```python
from build123d import *

# Parameters (mm, degrees)
SKETCH1_W           = 127.75
SKETCH1_H           = 298.45
SKETCH1_R           = 4.95
BOSS_EXTRUDE1_DEPTH = 10
SKETCH4_R           = 2.5
CUT_EXTRUDE2_DEPTH  = 11


with BuildPart() as part:
    # Sketch1 → Boss-Extrude1 (new body)
    with BuildSketch(Plane(origin=(0, 0, 0), x_dir=(1, 0, 0), z_dir=(0, 1, 0))):
        with Locations((63.875, 149.225)):
            Rectangle(SKETCH1_W, SKETCH1_H)
        with Locations((19, 277)):
            Circle(SKETCH1_R, mode=Mode.SUBTRACT)
        with Locations((108.75, 277)):
            Circle(SKETCH1_R, mode=Mode.SUBTRACT)
        with Locations((108.75, 19)):
            Circle(SKETCH1_R, mode=Mode.SUBTRACT)
        with Locations((19, 19)):
            Circle(SKETCH1_R, mode=Mode.SUBTRACT)
        with Locations((19, 108)):
            Circle(SKETCH1_R, mode=Mode.SUBTRACT)
        with Locations((108.75, 108)):
            Circle(SKETCH1_R, mode=Mode.SUBTRACT)
        with Locations((19, 188)):
            Circle(SKETCH1_R, mode=Mode.SUBTRACT)
        with Locations((108.75, 188)):
            Circle(SKETCH1_R, mode=Mode.SUBTRACT)
    extrude(amount=BOSS_EXTRUDE1_DEPTH)

    # Sketch4 → Cut-Extrude2 (cut, through all)
    with BuildSketch(Plane(origin=(0, 10, 0), x_dir=(1, 0, 0), z_dir=(0, 1, 0))):
        with Locations((93.875, 267.45)):
            Circle(SKETCH4_R)
        with Locations((33.875, 267.45)):
            Circle(SKETCH4_R)
        with Locations((93.875, 53.1375)):
            Circle(SKETCH4_R)
        with Locations((33.875, 53.1375)):
            Circle(SKETCH4_R)
    extrude(amount=-CUT_EXTRUDE2_DEPTH, mode=Mode.SUBTRACT)


solid = part.part
```
Work out the finished part from the listing and answer in its coordinate system (mm). Round coordinates to 2 decimals unless told otherwise and drop trailing zeros. Write each loop counter-clockwise with the first axis right and the second up, starting at its lowest first coordinate (ties: lowest second). Pieces come first, ordered by that corner, then holes.
1) A cutting plane is placed at A-A on z = -108. Determine the outline of the cut face in (x, y), and give its area (3 significant figures).
2) A cutting plane is placed at B-B on x = 108.75. Determine the outline of the cut face in (y, z).
3) Determine the mould class of faces 1 (the face through (127.75, 5, -147)), 2 (the face through (17.927, 4.93, -183.168)), 3 (the face through (63, 5, 0)) for opening direction Z: pulls with the +Z half, pulls with the -Z half, needs draft (parallel to the pull), parting line crosses it, or undercut.
4) A flat-ended cylindrical pin translates along its axis: P1, Ø6, axis at x = 108.75, z = -108, coming from the +Y side. Find the tip coordinate at first contact, or state that the pin passes through.
5) Consider probe 1 along X at (y, z) = (4.5, -108); probe 2 along Z at (x, y) = (108.75, 3.5); probe 3 along X at (y, z) = (1, -265.5). Determine where each line is inside the solid, lowest interval first.
6) A cutting plane is placed at C-C on y = 4. Give the number of separate pieces and of enclosed holes in the cut face, and give its area (3 significant figures).
Entries:
1. outline: (0, 0) - (14.05, 0) - (14.05, 10) - (0, 10) - close; (23.95, 0) - (103.8, 0) - (103.8, 10) - (23.95, 10) - close; (113.7, 0) - (127.75, 0) - (127.75, 10) - (113.7, 10) - close
1. area: 1,080 mm2
2. outline: (0, -298.45) - (10, -298.45) - (10, -281.95) - (0, -281.95) - close; (0, -272.05) - (10, -272.05) - (10, -192.95) - (0, -192.95) - close; (0, -183.05) - (10, -183.05) - (10, -112.95) - (0, -112.95) - close; (0, -103.05) - (10, -103.05) - (10, -23.95) - (0, -23.95) - close; (0, -14.05) - (10, -14.05) - (10, 0) - (0, 0) - close
3. face 1: needs draft
3. face 2: undercut
3. face 3: pulls with the +Z half
4. P1: passes through
5. probe 1: x = 0 to 14.05, 23.95 to 103.8, 113.7 to 127.75
5. probe 2: z = -298.45 to -281.95, -272.05 to -192.95, -183.05 to -112.95, -103.05 to -23.95, -14.05 to 0
5. probe 3: x = 0 to 32.31, 35.44 to 92.31, 95.44 to 127.75
6. separate pieces: 1
6. enclosed holes: 12
6. area: 37,400 mm2
